Build history of the part. All positions in model axes, mm. A direction names the side the tool comes from. Round coordinates to 2 decimals unless told otherwise and drop trailing zeros. Loops run counter-clockwise (first coordinate to the right, second up) from the corner with the lowest first, then second, coordinate; pieces in that order, holes last. Notation, with made-up numbers: M -5.5,-9 L 19.5,-9 A10 ccw 19.5,0 Z; hole C -35,83 d3. An arc over 180 degrees is marked long. Write each question's results on one line, items separated by ' | '. Start each with the question number.
```python
from build123d import *

# Parameters (mm, degrees)
SKETCH1_W             = 5.08
SKETCH1_H             = 19.05
BOSS_EXTRUDE1_DEPTH   = 35
F_5_0MM_DOWEL_HOLE1_D = 5.3
F_5_0MM_DOWEL_HOLE2_D = 5.3


with BuildPart() as part:
    # Sketch1 → Boss-Extrude1 (new body)
    with BuildSketch(Plane.XY):
        Polygon((0, 2.54), (0, 0), (17.78, 0), (17.78, 2.54), (5.08, 2.54), align=None)
        with Locations((2.54, 12.065)):
            Rectangle(SKETCH1_W, SKETCH1_H)
    extrude(amount=BOSS_EXTRUDE1_DEPTH)

    # Ø5.0mm Dowel Hole1 (through all)
    with Locations(Plane(origin=(5.08, 0, 0), x_dir=(0, 0, -1), z_dir=(1, 0, 0))):
        with Locations((-30, 15.24), (-5, 15.24)):
            Hole(F_5_0MM_DOWEL_HOLE1_D / 2)

    # Ø5.0mm Dowel Hole2 (through all)
    with Locations(Plane(origin=(0, 2.54, 0), x_dir=(1, 0, 0), z_dir=(0, 1, 0))):
        with Locations((11.43, -27.38), (11.43, -7.62)):
            Hole(F_5_0MM_DOWEL_HOLE2_D / 2)


solid = part.part
```
Item 1: Tool access for faces 4 (the flat face through (17.78, 1, 17)), 5 (the flat face through (5.08, 12, 17)): list every direction of +Z, -Z, +X, -X, +Y, -Y with a clear straight run to the whole face (end or side of a thin tool).
Item 2: Saw through at B-B, the plane x = 11. Give the cut face in (y, z), then the cut area to 3 significant figures.
Item 3: Drop flat-ended pins along their axis: pin 1 (6.5 mm diameter, centred on x = 12.5, z = 15, fed in from +Y); pin 2 (6 mm diameter, centred on y = 4.5, z = 18, fed in from +X); pin 3 (3 mm diameter, centred on y = 15.24, z = 30, fed in from +X). Give the stop position or say it passes through.
Item 4: Drill centre lines: line 1 along Z through (x, y) = (11.43, 1.3); line 2 along Z through (x, y) = (1.75, 13); line 3 along X through (y, z) = (2.05, 27.38). Where is each one in solid material? Low to high. Write a range as [from, to].
Item 5: Saw through at A-A, the plane y = 15.24. Give the cut face in (x, z), then the cut area to 3 significant figures.
Item 6: Saw through at D-D, the plane x = 8.25. Give the cut face in (y, z), then the cut area to 3 significant figures.
Item 7: Mould opens along Z. For faces 1 (the flat face through (9, 0, 17)), 2 (the cylindrical face through (13.533, 1.252, 9.232)), 3 (the flat face through (4.8, 8.5, 35)) say: released by +Z, released by -Z, zero draft, split by the parting line, or undercut.
Item 8: Saw through at C-C, the plane z = 23.5. Give the cut face in (x, y).
Working result:
1) face 4: +Z, -Z, +X, +Y, -Y | face 5: +Z, -Z, +X, +Y
2) outline: M 0,0 L 2.54,0 L 2.54,5.01 L 0,5.01 Z; M 0,10.23 L 2.54,10.23 L 2.54,24.77 L 0,24.77 Z; M 0,29.99 L 2.54,29.99 L 2.54,35 L 0,35 Z | area: 62.3 mm²
3) pin 1: stops at y = 2.54 | pin 2: stops at x = 17.78 | pin 3: passes through
4) line 1: z = [0, 4.97], [10.27, 24.73], [30.03, 35] | line 2: z = [0, 3.58], [6.42, 28.58], [31.42, 35] | line 3: x = [0, 8.78], [14.08, 17.78]
5) outline: M 0,0 L 5.08,0 L 5.08,2.35 L 0,2.35 Z; M 0,7.65 L 5.08,7.65 L 5.08,27.35 L 0,27.35 Z; M 0,32.65 L 5.08,32.65 L 5.08,35 L 0,35 Z | area: 124 mm²
6) outline: M 0,0 L 2.54,0 L 2.54,35 L 0,35 Z | area: 88.9 mm²
7) face 1: zero draft | face 2: undercut | face 3: released by +Z
8) outline: M 0,0 L 17.78,0 L 17.78,2.54 L 5.08,2.54 L 5.08,21.59 L 0,21.59 Z
